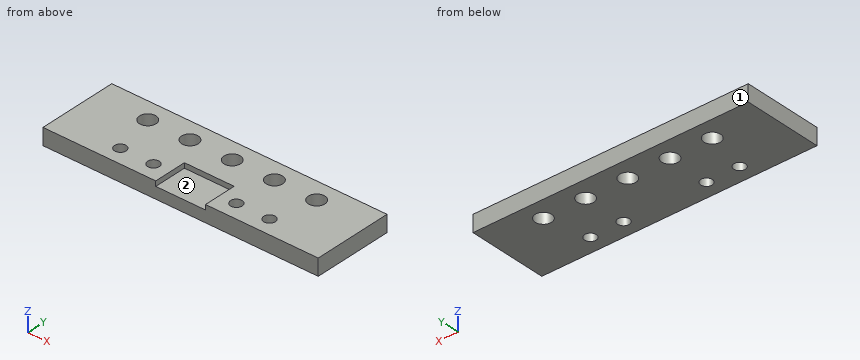
from build123d import *

# Parameters (mm, degrees)
F0_W      = 65
F0_H      = 10
F1_DEPTH  = 10
F2_W      = 15
F2_H      = 10
F3_DEPTH  = 3
F2_R      = 1.75
F4_DEPTH  = 25
F5_DEPTH  = 9
F6_DEPTH  = 9
F7_DEPTH  = 5
F8_DEPTH  = 1.5
F9_W      = 83
F9_H      = 5
F10_DEPTH = 14
F11_R     = 2.5
F12_DEPTH = 25


with BuildPart() as f1:
    # F0 (on Top) → F1 (new body)
    with BuildSketch(Plane.XY):
        Rectangle(F0_W, F0_H)
    extrude(amount=F1_DEPTH)

    # F2 (on face) → F3 (cut)
    with BuildSketch(Plane.XY.offset(10)):
        Rectangle(F2_W, F2_H)
    extrude(amount=-F3_DEPTH, mode=Mode.SUBTRACT)

    # F2 (on face) → F4 (cut)
    with BuildSketch(Plane.XY.offset(10)):
        with Locations((-22.5, 0)):
            Circle(F2_R)
        with Locations((-12.5, 0)):
            Circle(F2_R)
        with Locations((12.5, 0)):
            Circle(F2_R)
        with Locations((22.5, 0)):
            Circle(F2_R)
    extrude(amount=-F4_DEPTH, mode=Mode.SUBTRACT)

    # F5 (add): a face of the model
    f5_faces = [f1.faces().sort_by_distance(p)[0] for p in [
        (32.5, 0, 5),
    ]]
    extrude(f5_faces, amount=F5_DEPTH)

    # F6 (add): a face of the model
    f6_faces = [f1.faces().sort_by_distance(p)[0] for p in [
        (-32.5, 0, 5),
    ]]
    extrude(f6_faces, amount=F6_DEPTH)

    # F7 (cut): a face of the model
    f7_faces = [f1.faces().sort_by_distance(p)[0] for p in [
        (0, 0, 0),
    ]]
    extrude(f7_faces, amount=-F7_DEPTH, mode=Mode.SUBTRACT)

    # F8 (add): a face of the model
    f8_faces = [f1.faces().sort_by_distance(p)[0] for p in [
        (0, 0, 7),
    ]]
    extrude(f8_faces, amount=F8_DEPTH)

    # F9 (on face) → F10 (join)
    with BuildSketch(Plane(origin=(0, 5, 0), x_dir=(-1, 0, 0), z_dir=(0, 1, 0))):
        with Locations((0, 7.5)):
            Rectangle(F9_W, F9_H)
    extrude(amount=F10_DEPTH)

    # F11 (on face) → F12 (cut)
    with BuildSketch(Plane.XY.offset(10)):
        with Locations((12.73, 13)):
            Circle(F11_R)
        with Locations((25.46, 13)):
            Circle(F11_R)
        with Locations((0, 13)):
            Circle(F11_R)
        with Locations((-12.73, 13)):
            Circle(F11_R)
        with Locations((-25.46, 13)):
            Circle(F11_R)
    extrude(amount=-F12_DEPTH, mode=Mode.SUBTRACT)


solid = f1.part
Could you check a few things on this model? Use its own coordinates, in mm. Face numbers are marked on the shaded views. Give positions to 0.01 mm unless a question says otherwise; leave off trailing zeros. Order: outer loops, then holes, each group sorted by start corner. A loop starts at its lowest first (then second) coordinate and runs counter-clockwise, first axis right, second up. Notation, with made-up numbers: (73, -28.5) - (123, -28.5) arc R20 ccw to (123, 8.5) - close; hole circle Ø4 at (71, 49). An arc over 180 degrees is marked (long way). One line per item, written item: value. Start each with the question number.
1. Imagine slicing it at A-A on y = 13. List the corners of the cut face in (x, z) for me, plus the area to 3 significant figures.
2. Imagine slicing it at B-B on x = 0. List the corners of the cut face in (y, z) for me, plus the area to 3 significant figures.
3. Imagine slicing it at C-C on y = 0. List the corners of the cut face in (x, z) for me, plus the area to 4 significant figures.
4. Imagine slicing it at D-D on z = 7.8. Give the number of separate pieces and of enclosed holes in the cut face, plus the area to 3 significant figures.
5. If I drill on probe 1 along Y at (x, z) = (-12.73, 6.15); probe 2 along Y at (x, z) = (25.46, 7.4); probe 3 along X at (y, z) = (2.5, 9.2), over which ranges is the centre line in solid material (lowest first)?
6. For P1, Ø1.2, axis at x = -1.5, z = 9.5, coming from the -Y side; P2, Ø6.5, axis at x = -12.73, y = 13, coming from the -Z side, each with a flat end and sliding along its axis, tell me the tip position at first contact or that it passes through.
7. Thinking about a two-plate mould opening in X: for the marked faces 1 and 2, which applies, +X half, -X half, draft (parallel to the pull), parting line (faces both ways), or undercut?
Values:
1. outline: (-41.5, 5) - (-27.96, 5) - (-27.96, 10) - (-41.5, 10) - close; (-22.96, 5) - (-15.23, 5) - (-15.23, 10) - (-22.96, 10) - close; (-10.23, 5) - (-2.5, 5) - (-2.5, 10) - (-10.23, 10) - close; (2.5, 5) - (10.23, 5) - (10.23, 10) - (2.5, 10) - close; (15.23, 5) - (22.96, 5) - (22.96, 10) - (15.23, 10) - close; (27.96, 5) - (41.5, 5) - (41.5, 10) - (27.96, 10) - close
1. area: 290 mm²
2. outline: (-5, 5) - (10.5, 5) - (10.5, 10) - (5, 10) - (5, 8.5) - (-5, 8.5) - close; (15.5, 5) - (19, 5) - (19, 10) - (15.5, 10) - close
2. area: 80.0 mm²
3. outline: (-41.5, 5) - (-24.25, 5) - (-24.25, 10) - (-41.5, 10) - close; (-20.75, 5) - (-14.25, 5) - (-14.25, 10) - (-20.75, 10) - close; (-10.75, 5) - (10.75, 5) - (10.75, 10) - (7.5, 10) - (7.5, 8.5) - (-7.5, 8.5) - (-7.5, 10) - (-10.75, 10) - close; (14.25, 5) - (20.75, 5) - (20.75, 10) - (14.25, 10) - close; (24.25, 5) - (41.5, 5) - (41.5, 10) - (24.25, 10) - close
3. area: 322.5 mm²
4. separate pieces: 1
4. enclosed holes: 9
4. area: 1,860 mm²
5. probe 1: -5 to -1.73, 1.73 to 10.5, 15.5 to 19
5. probe 2: -5 to 10.5, 15.5 to 19
5. probe 3: -41.5 to -7.5, 7.5 to 41.5
6. P1: y = 5
6. P2: z = 5
7. face 1: draft
7. face 2: undercut
